Job drawing, mm, ordinate dimensions from the low corner. One solid piece. Give positions to 0.01 mm unless a question says otherwise; leave off trailing zeros. Order: outer loops, then holes, each group sorted by start corner. A loop starts at its lowest first (then second) coordinate and runs counter-clockwise, first axis right, second up.
1. Slice it at D-D on z = 0.7. List the corners of the cut face in (x, y).
2. Mould opens along X. For the marked faces 1, 2 and 3 say: +X half, -X half, draft (parallel to the pull), parting line (faces both ways), or undercut.
3. Drop flat-ended pins along their axis: pin 1 Ø2 at (y, z) = (8.5, 1.5) entering from +X; pin 2 Ø2 at (x, z) = (26.5, 1.5) entering from -Y; pin 3 Ø9.5 at (x, y) = (21, 12.5) entering from +Z; pin 4 Ø1.5 at (x, z) = (30, 3) entering from +Y. Give the stop position or say it passes through.
4. Slice it at A-A on y = 17.5. List the corners of the cut face in (x, z), and give its area (3 significant figures).
5. Slice it at C-C on z = 3.6. List the corners of the cut face in (x, y).
6. Probe line 1 (X direction, y = 17.5, z = 2.95); line 2 (Y direction, x = 11.5, z = 3.8) (1 decimal); line 3 (X direction, y = 15.5, z = 0.45) (1 decimal). List the from-to ranges inside material, lowest first.
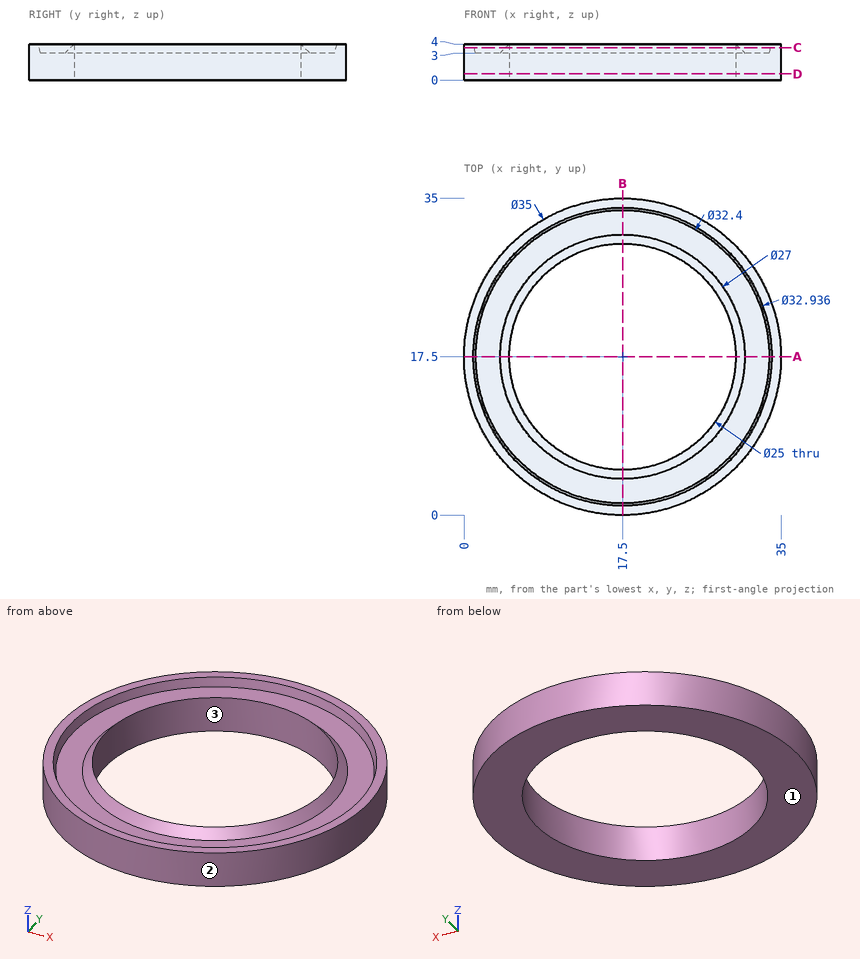
Data:
1. outline: circle Ø35 at (17.5, 17.5); hole circle Ø25 at (17.5, 17.5)
2. face 1: draft
2. face 2: parting line
2. face 3: undercut
3. pin 1: stops at x = 33.06
3. pin 2: stops at y = 1.94
3. pin 3: passes through
3. pin 4: stops at y = 30.47
4. outline: (0, 0) - (5, 0) - (5, 4) - (4, 3) - (1.3, 3) - (1.03, 4) - (0, 4) - close; (30, 0) - (35, 0) - (35, 4) - (33.97, 4) - (33.7, 3) - (31, 3) - (30, 4) - close
4. area: 33.3 mm2
5. outline: circle Ø35 at (17.5, 17.5); circle Ø25.8 at (17.5, 17.5); hole circle Ø32.72 at (17.5, 17.5); hole circle Ø25 at (17.5, 17.5)
6. line 1: x = 0 to 5, 30 to 35
6. line 2: y = 1.1 to 2.2, 6.3 to 6.5, 28.5 to 28.7, 32.8 to 33.9
6. line 3: x = 0.1 to 5.2, 29.8 to 34.9
